Build history of the part. All positions in model axes, mm. A direction names the side the tool comes from. Give positions to 0.01 mm unless a question says otherwise; leave off trailing zeros. Loops run counter-clockwise (first coordinate to the right, second up) from the corner with the lowest first, then second, coordinate; pieces in that order, holes last.
1) Wall check: line 1 (X direction, y = 21, z = 2.5); line 2 (Z direction, x = -5.35, y = 23); line 3 (Z direction, x = 0, y = 1.4). Give the ranges that are in metal, low to high.
2) Band-saw the part on D-D on x = 0. List the corners of the cut face in (y, z).
3) Two-plate mould, pull along Y, no slides. Class faces 5 (the cylindrical face through (-0.325, 1.972, 7.536)), 6 (the cylindrical face through (5.285, 7.93, 17.699)), 7 (the cylindrical face through (8.43, 15.4, 9.11)): +Y half, -Y half, draft (parallel to the pull), parting line (faces both ways), or undercut.
4) Band-saw the part on C-C on y = 23. List the corners of the cut face in (x, z).
5) Flat gauge pins, fed straight in: P1, Ø5, axis at y = 24.5, z = 11, coming from the -X side; P2, Ø6.5, axis at y = 23, z = 9, coming from the +X side; P3, Ø1.5, axis at y = 15.5, z = 2.5, coming from the +X side. Where does each tip first touch, or does it go through?
6) Band-saw the part on B-B on z = 9. State how many separate pieces and enclosed holes the cut face has, then the cut area to 3 significant figures.
7) 3-axis set-ups, long thin cutter, end or side, ignore diameter. For faces 1 (the cylindrical face through (-5.965, 19.563, 0.301)), 2 (the flat face through (-5, 8, 9)), 3 (the cylindrical face through (4.151, 12.301, 0.285)), 4 (the cylindrical face through (-5.965, 19.437, 17.699)): which of +Z, -Z, +X, -X, +Y, -Y reach the whole face in a straight line?
8) Band-saw the part on A-A on y = 9. List the corners of the cut face in (x, z), then the cut area to 3 significant figures.
```python
from build123d import *

# Parameters (mm, degrees)
PAD_DEPTH       = 18
SKETCH002_R     = 2.5
POCKET_DEPTH    = 15.251
SKETCH003_R     = 1.5
POCKET001_DEPTH = 30.001
FILLET_R        = 2
FILLET001_R     = 6
FILLET002_R     = 1


with BuildPart() as part:
    # Sketch → Pad (new body)
    with BuildSketch(Plane.XY):
        Polygon((-9, 0), (9, 0), (9, 16), (6.25, 16), (6.25, 30), (2.25, 30), (2.25, 12), (5, 12), (5, 4), (-5, 4), (-5, 12), (-2.25, 12), (-2.25, 30), (-6.25, 30), (-6.25, 16), (-9, 16), align=None)
    extrude(amount=PAD_DEPTH)

    # Sketch002 (on Face15 of Pad) → Pocket (cut, through all)
    with BuildSketch(Plane(origin=(-6.25, 0, 0), x_dir=(0, -1, 0), z_dir=(-1, 0, 0))):
        with Locations((-23, 9)):
            Circle(SKETCH002_R)
    extrude(amount=-POCKET_DEPTH, mode=Mode.SUBTRACT)

    # Sketch003 (on Face2 of Pocket) → Pocket001 (cut, through all)
    with BuildSketch(Plane.XZ):
        with Locations((0, 9)):
            Circle(SKETCH003_R)
    extrude(amount=-POCKET001_DEPTH, mode=Mode.SUBTRACT)

    # Fillet
    fillet_edges = [part.edges().sort_by_distance(p)[0] for p in [
        (-9, 16, 9),
        (9, 16, 9),
    ]]
    fillet(fillet_edges, radius=FILLET_R)

    # Fillet001
    fillet001_edges = [part.edges().sort_by_distance(p)[0] for p in [
        (4.25, 30, 0),
        (-4.25, 30, 0),
        (4.25, 30, 18),
        (-4.25, 30, 18),
    ]]
    fillet(fillet001_edges, radius=FILLET001_R)

    # Fillet002
    fillet002_edges = [part.edges().sort_by_distance(p)[0] for p in [
        (-6.25, 20, 18),
        (-4.25, 24, 18),
        (-6.625, 16, 18),
        (-2.25, 18, 18),
        (-8.414214, 15.414214, 18),
        (-3.625, 12, 18),
        (-9, 7, 18),
        (-5, 8, 18),
        (0, 0, 18),
        (0, 4, 18),
        (9, 7, 18),
        (5, 8, 18),
        (8.414214, 15.414214, 18),
        (3.625, 12, 18),
        (6.625, 16, 18),
        (2.25, 18, 18),
        (6.25, 20, 18),
        (4.25, 24, 18),
        (-6.25, 20, 0),
        (-4.25, 24, 0),
        (-6.625, 16, 0),
        (-2.25, 18, 0),
        (-8.414214, 15.414214, 0),
        (-3.625, 12, 0),
        (-9, 7, 0),
        (-5, 8, 0),
        (0, 0, 0),
        (0, 4, 0),
        (9, 7, 0),
        (5, 8, 0),
        (8.414214, 15.414214, 0),
        (3.625, 12, 0),
        (6.625, 16, 0),
        (2.25, 18, 0),
        (6.25, 20, 0),
        (4.25, 24, 0),
    ]]
    fillet(fillet002_edges, radius=FILLET002_R)


solid = part.part
```
Findings below:
1. line 1: x = -6.25 to -2.25, 2.25 to 6.25
1. line 2: z = 0.01 to 6.5, 11.5 to 17.99
1. line 3: z = 0 to 7.5, 10.5 to 18
2. outline: (0, 1) arc R1 ccw to (1, 0) - (3, 0) arc R1 ccw to (4, 1) - (4, 7.5) - (0, 7.5) - close; (0, 10.5) - (4, 10.5) - (4, 17) arc R1 ccw to (3, 18) - (1, 18) arc R1 ccw to (0, 17) - close
3. face 5: draft
3. face 6: undercut
3. face 7: +Y half
4. outline: (-6.25, 1) arc R1 ccw to (-5.25, 0) - (-3.25, 0) arc R1 ccw to (-2.25, 1) - (-2.25, 6.5) - (-6.25, 6.5) - close; (-6.25, 11.5) - (-2.25, 11.5) - (-2.25, 17) arc R1 ccw to (-3.25, 18) - (-5.25, 18) arc R1 ccw to (-6.25, 17) - close; (2.25, 1) arc R1 ccw to (3.25, 0) - (5.25, 0) arc R1 ccw to (6.25, 1) - (6.25, 6.5) - (2.25, 6.5) - close; (2.25, 11.5) - (6.25, 11.5) - (6.25, 17) arc R1 ccw to (5.25, 18) - (3.25, 18) arc R1 ccw to (2.25, 17) - close
5. P1: stops at x = -6.25
5. P2: stops at x = 6.25
5. P3: stops at x = 8.85
6. separate pieces: 4
6. enclosed holes: 0
6. area: 247 mm2
7. face 1: -Z, -X, +Y
7. face 2: +Z, -Z
7. face 3: -Z
7. face 4: +Z, -X, +Y
8. outline: (-9, 1) arc R1 ccw to (-8, 0) - (-6, 0) arc R1 ccw to (-5, 1) - (-5, 17) arc R1 ccw to (-6, 18) - (-8, 18) arc R1 ccw to (-9, 17) - close; (5, 1) arc R1 ccw to (6, 0) - (8, 0) arc R1 ccw to (9, 1) - (9, 17) arc R1 ccw to (8, 18) - (6, 18) arc R1 ccw to (5, 17) - close
8. area: 142 mm2
